```python
from build123d import *

# Parameters (mm, degrees)
SKETCH1_W           = 155.702807198
SKETCH1_H           = 58
SKETCH1_R           = 1.5
BOSS_EXTRUDE2_DEPTH = 5
SKETCH2_R           = 1
BOSS_EXTRUDE3_DEPTH = 5
SKETCH3_R           = 1.5
SKETCH3_R_2         = 1
BOSS_EXTRUDE4_DEPTH = 5


with BuildPart() as part:
    # Sketch1 → Boss-Extrude2 (new body)
    with BuildSketch(Plane(origin=(0, 0, 0), x_dir=(1, 0, 0), z_dir=(0, 1, 0))):
        with Locations((1.171695753, -5)):
            Rectangle(SKETCH1_W, SKETCH1_H)
        Polygon((-76.679707846, 44), (-76.679707846, 24), (79.023099352, 24), (79.023099352, 44), (62.885457038, 44), (59.885457038, 44), (-57.542065533, 44), (-60.542065533, 44), align=None)
        with Locations((-59.042065533, 34)):
            Circle(SKETCH1_R, mode=Mode.SUBTRACT)
        with Locations((61.385457038, 34)):
            Circle(SKETCH1_R, mode=Mode.SUBTRACT)
        Polygon((-76.679707846, -44), (-60.542065533, -44), (-57.542065533, -44), (59.885457038, -44), (62.885457038, -44), (79.023099352, -44), (79.023099352, -34), (-76.679707846, -34), align=None)
        with Locations((-59.042065533, -39)):
            Circle(SKETCH1_R, mode=Mode.SUBTRACT)
        with Locations((61.385457038, -39)):
            Circle(SKETCH1_R, mode=Mode.SUBTRACT)
    extrude(amount=BOSS_EXTRUDE2_DEPTH)

    # Sketch2 → Boss-Extrude3 (add)
    with BuildSketch(Plane(origin=(0, 5, 0), x_dir=(1, 0, 0), z_dir=(0, 1, 0))):
        Polygon((-23.828304247, 44), (26.171695753, 44), (26.171695753, 50.823606938), (13.671695753, 56.49492606), (-11.328304247, 56.49492606), (-23.828304247, 50.823606938), align=None)
        with Locations((1.171695753, 50.24746303)):
            Circle(SKETCH2_R, mode=Mode.SUBTRACT)
    extrude(amount=-BOSS_EXTRUDE3_DEPTH)

    # Sketch3 → Boss-Extrude4 (add)
    with BuildSketch(Plane(origin=(0, 5, 0), x_dir=(1, 0, 0), z_dir=(0, 1, 0))):
        with Locations((61.385457038, 34)):
            Circle(SKETCH3_R)
        with Locations((61.385457038, 34)):
            Circle(SKETCH3_R_2, mode=Mode.SUBTRACT)
        with Locations((61.385457038, -39)):
            Circle(SKETCH3_R)
        with Locations((61.385457038, -39)):
            Circle(SKETCH3_R_2, mode=Mode.SUBTRACT)
        with Locations((-59.042065533, -39)):
            Circle(SKETCH3_R)
        with Locations((-59.042065533, -39)):
            Circle(SKETCH3_R_2, mode=Mode.SUBTRACT)
        with Locations((-59.042065533, 34)):
            Circle(SKETCH3_R)
        with Locations((-59.042065533, 34)):
            Circle(SKETCH3_R_2, mode=Mode.SUBTRACT)
    extrude(amount=-BOSS_EXTRUDE4_DEPTH)


solid = part.part
```
Verification items for the finished model (mm, model axes). A direction names the side the tool comes from. Coordinates: 2 decimals unless noted, no trailing zeros. Loops run counter-clockwise (first coordinate to the right, second up) from the corner with the lowest first, then second, coordinate; pieces in that order, holes last. Notation, with made-up numbers: (32, -25) -> (90, -25) arc R9 cw to (90, -10) -> close; hole circle Ø11 at (51, 4). An arc over 180 degrees is marked (long way). Answer in a Markdown table with one row per item. Add a question column.
1. Access from +Z, -Z, +X, -X, +Y, -Y to the whole of each face (thin tool, end or side, straight path). Record for faces 1 (the face through (-23.828, 3, -47)), 2 (the face through (26.172, 3, -47)), 3 (the face through (0, 0, -7)).
2. Section check C-C, the plane x = 44.5. Enter the section's corners in (y, z), then the cut area to 3 significant figures.
3. Material ranges on probe 1 along X at (y, z) = (3.95, 39); probe 2 along Z at (x, y) = (-37.5, 3.35); probe 3 along X at (y, z) = (4.1, -46), recorded low to high. Write a range as [from, to].
4. Section check A-A, the plane y = 1. Enter the section's corners in (x, z).
5. Depth check by flat-ended pin: P1, Ø2.5, axis at x = -51, y = 2, coming from the -Z side; P2, Ø1.5, axis at y = 2.5, z = -46.5, coming from the -X side; P3, Ø1.5, axis at y = 1.5, z = -46.5, coming from the +X side. Enter the tip coordinate at first touch or a pass-through.
6. Section check B-B, the plane z = -47. Enter the section's corners in (x, y), then the cut area to 3 significant figures.
Derived:
| question | item | result |
|---|---|---|
| 1 | face 1 | -Z, -X, +Y, -Y |
| 1 | face 2 | -Z, +X, +Y, -Y |
| 1 | face 3 | +Z, -Z, +X, -X, -Y |
| 2 | outline | (0, -44) -> (5, -44) -> (5, 44) -> (0, 44) -> close |
| 2 | area | 440 mm² |
| 3 | probe 1 | x = [-76.68, -60.04], [-58.04, 60.39], [62.39, 79.02] |
| 3 | probe 2 | z = [-44, 44] |
| 3 | probe 3 | x = [-23.83, 26.17] |
| 4 | outline | (-76.68, -44) -> (-23.83, -44) -> (-23.83, -50.82) -> (-11.33, -56.49) -> (13.67, -56.49) -> (26.17, -50.82) -> (26.17, -44) -> (79.02, -44) -> (79.02, 44) -> (-76.68, 44) -> close; hole circle Ø2 at (-59.04, -34); hole circle Ø2 at (-59.04, 39); hole circle Ø2 at (1.17, -50.25); hole circle Ø2 at (61.39, -34); hole circle Ø2 at (61.39, 39) |
| 5 | P1 | stops at z = -44 |
| 5 | P2 | stops at x = -23.83 |
| 5 | P3 | stops at x = 26.17 |
| 6 | outline | (-23.83, 0) -> (26.17, 0) -> (26.17, 5) -> (-23.83, 5) -> close |
| 6 | area | 250 mm² |
